For this review, take the finished solid that the model builds, in its own axes (mm). Face numbers are marked on the shaded views. A direction names the side the tool comes from. Coordinates: 2 decimals unless noted, no trailing zeros. Loops run counter-clockwise (first coordinate to the right, second up) from the corner with the lowest first, then second, coordinate; pieces in that order, holes last.
```python
from build123d import *

# Parameters (mm, degrees)
BOSS_EXTRUDE1_DEPTH        = 10
CUT_EXTRUDE1_DEPTH         = 5
F_3_1_3_1_DIAMETER_HOLE2_D = 3.1
BOSS_EXTRUDE2_DEPTH        = 10
FILLET1_R                  = 3
FILLET2_R                  = 2
SKETCH21_R                 = 2.1
CUT_EXTRUDE2_DEPTH         = 36.312840879
SKETCH22_R                 = 3.5
CUT_EXTRUDE3_DEPTH         = 2.5
CUT_EXTRUDE4_DEPTH         = 2.7
CUT_EXTRUDE4_DEPTH_BACK    = 0.2
SKETCH23_R                 = 2.5
SKETCH24_W                 = 2.5
SKETCH24_H                 = 3.5
SKETCH25_R                 = 2.5
CUT_EXTRUDE5_DEPTH         = 9.733021807
CUT_EXTRUDE6_DEPTH         = 2.5


with BuildPart() as part:
    # Sketch1 → Boss-Extrude1 (new body)
    with BuildSketch(Plane(origin=(0, 0, 0), x_dir=(1, 0, 0), z_dir=(0, 1, 0))):
        with BuildLine():
            ThreePointArc((-187.660784713, 29.722548358), (-190, 0), (-187.660784713, -29.722548358))
            Line((-187.660784713, -29.722548358), (-197.537668119, -31.286893008))
            ThreePointArc((-197.537668119, -31.286893008), (-200, 0), (-197.537668119, 31.286893008))
            Line((-197.537668119, 31.286893008), (-187.660784713, 29.722548358))
        make_face()
        with BuildLine():
            ThreePointArc((-197.537668119, -31.286893008), (-200, 0), (-197.537668119, 31.286893008))
            Line((-197.537668119, 31.286893008), (-200.500733141, 31.756196403))
            ThreePointArc((-200.500733141, 31.756196403), (-203, 0), (-200.500733141, -31.756196403))
            Line((-200.500733141, -31.756196403), (-197.537668119, -31.286893008))
        make_face()
        with BuildLine():
            Line((-184.697719691, 29.253244963), (-187.660784713, 29.722548358))
            ThreePointArc((-187.660784713, 29.722548358), (-190, 0), (-187.660784713, -29.722548358))
            Line((-187.660784713, -29.722548358), (-184.697719691, -29.253244963))
            ThreePointArc((-184.697719691, -29.253244963), (-187, 0), (-184.697719691, 29.253244963))
        make_face()
    extrude(amount=BOSS_EXTRUDE1_DEPTH)

    # Sketch15 → Cut-Extrude1 (cut)
    with BuildSketch(Plane(origin=(0, 10, 0), x_dir=(1, 0, 0), z_dir=(0, 1, 0))):
        with BuildLine():
            Line((-199.749843554, 10), (-189.73665961, 10))
            ThreePointArc((-189.73665961, 10), (-188.956218405, 19.88837666), (-187.660784713, 29.722548358))
            Line((-187.660784713, 29.722548358), (-197.537668119, 31.286893008))
            ThreePointArc((-197.537668119, 31.286893008), (-198.928692466, 20.673057674), (-199.749843554, 10))
        make_face()
        with BuildLine():
            ThreePointArc((-187.660784713, -29.722548358), (-188.956218405, -19.88837666), (-189.73665961, -10))
            Line((-189.73665961, -10), (-199.749843554, -10))
            ThreePointArc((-199.749843554, -10), (-198.928692466, -20.673057674), (-197.537668119, -31.286893008))
            Line((-197.537668119, -31.286893008), (-187.660784713, -29.722548358))
        make_face()
    extrude(amount=-CUT_EXTRUDE1_DEPTH, mode=Mode.SUBTRACT)

    # Ø3.1 (3.1) Diameter Hole2 (through all)
    with Locations(Plane(origin=(0, 0, 0), x_dir=(-1, 0, 0), z_dir=(0, -1, 0))):
        with Locations((193.331747968, -25.452607483), (194.257966128, -16.995369836), (194.257966128, 16.995369836), (193.331747968, 25.452607483)):
            Hole(F_3_1_3_1_DIAMETER_HOLE2_D / 2)

    # Sketch19 → Boss-Extrude2 (add)
    with BuildSketch(Plane(origin=(0, 0, 0), x_dir=(1, 0, 0), z_dir=(0, 1, 0))):
        with BuildLine():
            Line((-185.102830261, -12.132280472), (-186.599618646, -12.230385166))
            ThreePointArc((-186.599618646, -12.230385166), (-187, 0), (-186.599618646, 12.230385166))
            Line((-186.599618646, 12.230385166), (-185.102830261, 12.132280472))
            ThreePointArc((-185.102830261, 12.132280472), (-185.5, 0), (-185.102830261, -12.132280472))
        make_face()
    extrude(amount=BOSS_EXTRUDE2_DEPTH)

    # Fillet1
    # the kernel refuses this fillet: 3 mm, written as the material it adds along each edge
    with BuildSketch(Plane(origin=(-186.599618646, 0, -12.230385166), x_dir=(0.07241784502459461, 0, -0.9973743809232287), z_dir=(0, 1, 0))) as fillet1_piece_1:
        with BuildLine():
            CenterArc((2.608644701, -2.999925838), FILLET1_R, 89.597127862, 60.403689883)
            Line((0.010547081, -1.499962919), (-0.041414871, -1.469963661))
            ThreePointArc((-0.041414871, -1.469963661), (-0.054724976, -0.750403343), (-0.059998517, -0.000421883))
            Line((-0.059998517, -0.000421883), (-0.000421883, 0.059998517))
            ThreePointArc((-0.000421883, 0.059998517), (1.314869431, 0.064622735), (2.630160746, 0.059998517))
            Line((2.630160746, 0.059998517), (2.629738863, 0))
        make_face()
    extrude(amount=10)
    with BuildSketch(Plane(origin=(-186.599618646, 0, 12.230385166), x_dir=(0.0724178450245846, 0, 0.9973743809232295), z_dir=(0, 1, 0))) as fillet1_piece_2:
        with BuildLine():
            CenterArc((2.608644701, 2.999925838), FILLET1_R, 209.999182255, 60.403689883)
            Line((0.010547081, 1.499962919), (-0.041414871, 1.469963661))
            ThreePointArc((-0.041414871, 1.469963661), (-0.054724976, 0.750403343), (-0.059998517, 0.000421883))
            Line((-0.059998517, 0.000421883), (-0.000421883, -0.059998517))
            ThreePointArc((-0.000421883, -0.059998517), (1.314869431, -0.064622735), (2.630160746, -0.059998517))
            Line((2.630160746, -0.059998517), (2.629738863, 0))
        make_face()
    extrude(amount=10)

    # Fillet2
    fillet2_edges = [part.edges().sort_by_distance(p)[0] for p in [
        (-200.500733141, 5, 31.756196403),
        (-200.500733141, 5, -31.756196403),
        (-184.697719691, 5, -29.253244963),
        (-184.697719691, 5, 29.253244963),
    ]]
    fillet(fillet2_edges, radius=FILLET2_R)

    # Sketch21 → Cut-Extrude2 (cut, through all)
    with BuildSketch(Plane(origin=(-197.5, 0, 0), x_dir=(0, 0, -1), z_dir=(1, 0, 0))):
        with Locations((0, 10)):
            Circle(SKETCH21_R)
    extrude(amount=CUT_EXTRUDE2_DEPTH, mode=Mode.SUBTRACT)

    # Sketch22 → Cut-Extrude3 (cut)
    with BuildSketch(Plane(origin=(-197.5, 0, 0), x_dir=(0, 0, -1), z_dir=(1, 0, 0))):
        with Locations((0, 10)):
            Circle(SKETCH22_R)
    extrude(amount=CUT_EXTRUDE3_DEPTH, mode=Mode.SUBTRACT)

    # Sketch23 → Cut-Extrude4 (cut, two sides: drawn at the far end of the back side and taken through both)
    with BuildSketch(Plane(origin=(-197.5, 0, 0), x_dir=(0, 0, -1), z_dir=(1, 0, 0)).offset(-CUT_EXTRUDE4_DEPTH_BACK)):
        with Locations((0, 10)):
            Circle(SKETCH23_R)
    extrude(amount=CUT_EXTRUDE4_DEPTH + CUT_EXTRUDE4_DEPTH_BACK, mode=Mode.SUBTRACT)

    # Sketch24 → Cut-Revolve1 (revolve, cut)
    with BuildSketch(Plane(origin=(0, 10, 0), x_dir=(1, 0, 0), z_dir=(0, 1, 0))):
        with Locations((-186.716978193, 1.75)):
            Rectangle(SKETCH24_W, SKETCH24_H)
    revolve(axis=Axis((-185.5, 10, 0), (-1, 0, 0)), mode=Mode.SUBTRACT)

    # Sketch25 → Cut-Extrude5 (cut)
    with BuildSketch(Plane(origin=(-187.966978193, 0, 0), x_dir=(0, 0, -1), z_dir=(1, 0, 0))):
        with Locations((0, 10)):
            Circle(SKETCH25_R)
    extrude(amount=-CUT_EXTRUDE5_DEPTH, mode=Mode.SUBTRACT)

    # Sketch26 → Cut-Extrude6 (cut)
    with BuildSketch(Plane.XZ):
        with BuildLine():
            Line((-198.515528472, -31.441770873), (-186.662644351, -29.564458455))
            ThreePointArc((-186.662644351, -29.564458455), (-185.363721979, -28.773196969), (-184.996936421, -27.297133819))
            ThreePointArc((-184.996936421, -27.297133819), (-185.807261228, -21.087002508), (-186.409178624, -14.853219336))
            ThreePointArc((-186.409178624, -14.853219336), (-186.123110766, -13.316498702), (-185.102830261, -12.132280472))
            ThreePointArc((-185.102830261, -12.132280472), (-185.5, 0), (-185.102830261, 12.132280472))
            ThreePointArc((-185.102830261, 12.132280472), (-186.123110766, 13.316498702), (-186.409178624, 14.853219336))
            ThreePointArc((-186.409178624, 14.853219336), (-185.807261228, 21.087002508), (-184.996936421, 27.297133819))
            ThreePointArc((-184.996936421, 27.297133819), (-185.363721979, 28.773196969), (-186.662644351, 29.564458455))
            Line((-186.662644351, 29.564458455), (-198.515528472, 31.441770873))
            ThreePointArc((-198.515528472, 31.441770873), (-200.012003377, 31.078559473), (-200.806789416, 29.759592144))
            ThreePointArc((-200.806789416, 29.759592144), (-203, 0), (-200.806789416, -29.759592144))
            ThreePointArc((-200.806789416, -29.759592144), (-200.012003377, -31.078559473), (-198.515528472, -31.441770873))
        make_face()
    extrude(amount=-CUT_EXTRUDE6_DEPTH, mode=Mode.SUBTRACT)


solid = part.part
```
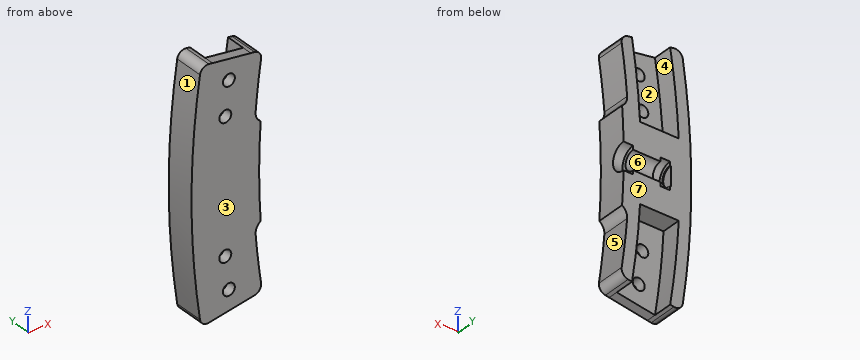
Q1. Machinability: for the marked faces 4, 5, 6 and 7, which of the approach directions +Z, -Z, +X, -X, +Y, -Y give a long, thin tool a straight path to every point of the face, cutting with its end or side? Answer none if there is none.
Q2. The part is to be moulded in two halves that separate along Z. For the marked faces 1, 2 and 3, say which applies: +Z half, -Z half, draft (parallel to the pull), parting line (faces both ways), or undercut.
Q3. Consider section A-A (y = 5.75). State the section outline as (x, z) points.
Q4. Consider section C-C (z = 0). State the section outline as (x, y) points.
Q5. For pin 1 Ø1.5 at (y, z) = (7, -0.5) entering from +X; pin 2 Ø3 at (y, z) = (8.5, 0) entering from +X; pin 3 Ø1.5 at (x, y) = (-197, 8.5) entering from -Z, all flat-tipped, find the tip position at first contact; note any pin that passes through.
Q6. Wall thickness on probe 1 along Z at (x, y) = (-186.75, 4); probe 2 along Y at (x, z) = (-192.5, -21); probe 3 along X at (y, z) = (9, 28): over which ranges is each line inside the solid? List them lowest first.
Q7. Consider section B-B (z = -18). State the section outline as (x, y) points.
Model answer:
1. face 4: +Y
1. face 5: +X, +Y, -Y
1. face 6: +X, +Y
1. face 7: +Z, -Z, +X, -X, +Y
2. face 1: parting line
2. face 2: undercut
2. face 3: draft
3. outline: (-200.81, -29.76) arc R2 ccw to (-198.52, -31.44) - (-197.54, -31.29) arc R200 cw to (-199.75, -10) - (-189.74, -10) arc R190 ccw to (-187.66, -29.72) - (-186.66, -29.56) arc R2 ccw to (-185, -27.3) arc R187 cw to (-186.41, -14.85) arc R3 cw to (-185.1, -12.13) arc R185.5 cw to (-185.1, 12.13) arc R3 cw to (-186.41, 14.85) arc R187 cw to (-185, 27.3) arc R2 ccw to (-186.66, 29.56) - (-187.66, 29.72) arc R190 ccw to (-189.74, 10) - (-199.75, 10) arc R200 cw to (-197.54, 31.29) - (-198.52, 31.44) arc R2 ccw to (-200.81, 29.76) arc R203 ccw to start
4. outline: (-203, 2.5) - (-185.5, 2.5) - (-185.5, 6.5) - (-187.97, 6.5) - (-187.97, 7.5) - (-195, 7.5) - (-195, 6.5) - (-197.5, 6.5) - (-197.5, 7.5) - (-197.7, 7.5) - (-197.7, 10) - (-203, 10) - close
5. pin 1: stops at x = -185.5
5. pin 2: stops at x = -187.97
5. pin 3: stops at z = -31.32
6. probe 1: z = -29.58 to 29.58
6. probe 2: y = 2.5 to 5
6. probe 3: x = -201.06 to -198.03, -187.93 to -185.02
7. outline: (-202.2, 2.5) - (-195.44, 2.5) - (-195.44, 5) - (-199.19, 5) - (-199.19, 10) - (-202.2, 10) - close; (-193.08, 2.5) - (-186.13, 2.5) - (-186.13, 10) - (-189.15, 10) - (-189.15, 5) - (-193.08, 5) - close
